Source: three-view drawing plus pictorial views. Frame: mm from the lowest corner of the part. Coordinates: 2 decimals unless noted, no trailing zeros. Loops run counter-clockwise (first coordinate to the right, second up) from the corner with the lowest first, then second, coordinate; pieces in that order, holes last. Notation, with made-up numbers: M -16,50.25 L 10,50.25 A18 ccw 10,80.25 Z; hole C 88.25,0.5 d1. An arc over 180 degrees is marked long. Use a Markdown table: item, result. Add a question column.
1. Line query: L1, parallel to X at y = 45.5, z = 75; L2, parallel to X at y = 27.5, z = 51.5; L3, parallel to Z at x = 90, y = 40.5. Output: solid intervals per line, ascending. Write a range as [from, to].
2. Pin query (flat end, axial travel): pin 1 (4 mm diameter, centred on y = 30, z = 3.5, fed in from -X); pin 2 (4 mm diameter, centred on x = 3, y = 20, fed in from -Z); pin 3 (8 mm diameter, centred on x = 5, z = 5, fed in from +Y). Return the tip coordinate at first contact, or that it passes through.
3. Section B-B on y = 22. Output: boundary loops of the cut face in (x, z), then the cut area to 3 significant figures.
4. Draft query along Z for the marked faces 1, 2, 3 and 4. Return one class per face: +Z half, -Z half, draft (parallel to the pull), parting line (faces both ways), or undercut.
5. Section A-A on z = 75. Output: boundary loops of the cut face in (x, y), then the cut area to 3 significant figures.
6. Section D-D on y = 45.5. Output: boundary loops of the cut face in (x, z), then the cut area to 3 significant figures.
7. Section C-C on x = 75. Output: boundary loops of the cut face in (y, z).
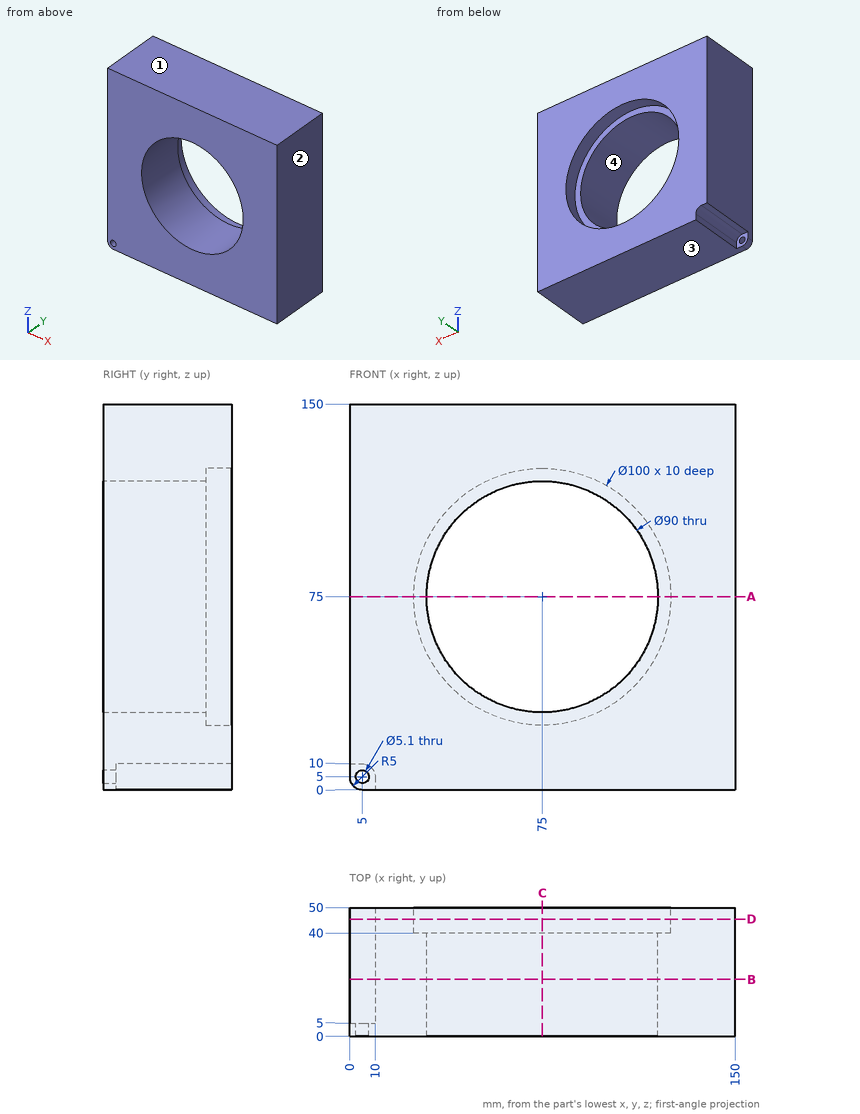
Answers below:
| question | item | result |
|---|---|---|
| 1 | L1 | x = [0, 25], [125, 150] |
| 1 | L2 | x = [0, 36.62], [113.38, 150] |
| 1 | L3 | z = [0, 27.3], [122.7, 150] |
| 2 | pin 1 | stops at x = 9.97 |
| 2 | pin 2 | stops at z = 10 |
| 2 | pin 3 | stops at y = 5 |
| 3 | outline | M 0,10 L 5,10 A5 cw 10,5 L 10,0 L 150,0 L 150,150 L 0,150 Z; hole C 75,75 d90 |
| 3 | area | 16,000 mm² |
| 4 | face 1 | +Z half |
| 4 | face 2 | draft |
| 4 | face 3 | -Z half |
| 4 | face 4 | undercut |
| 5 | outline | M 0,0 L 30,0 L 30,40 L 25,40 L 25,50 L 0,50 Z; M 120,0 L 150,0 L 150,50 L 125,50 L 125,40 L 120,40 Z |
| 5 | area | 2,900 mm² |
| 6 | outline | M 0,10 L 5,10 A5 cw 10,5 L 10,0 L 150,0 L 150,150 L 0,150 Z; hole C 75,75 d100 |
| 6 | area | 14,600 mm² |
| 7 | outline | M 0,0 L 50,0 L 50,25 L 40,25 L 40,30 L 0,30 Z; M 0,120 L 40,120 L 40,125 L 50,125 L 50,150 L 0,150 Z |
